```python
from build123d import *

# Parameters (mm, degrees)
BOSS_EXTRUDE6_DEPTH = 115
CUT_EXTRUDE5_START  = 2
SKETCH17_W          = 110
SKETCH17_H          = 71
CUT_EXTRUDE5_DEPTH  = 115
BOSS_EXTRUDE7_START = -12
BOSS_EXTRUDE7_DEPTH = 91
SKETCH22_R          = 3
SKETCH22_W          = 91
SKETCH22_H          = 3.970785373
CUT_EXTRUDE6_DEPTH  = 3.191306198
BOSS_EXTRUDE8_START = -12
SKETCH23_W          = 67.315835607
SKETCH23_H          = 18
BOSS_EXTRUDE8_DEPTH = 1
BOSS_EXTRUDE9_START = -12
SKETCH24_W          = 67.315835607
SKETCH24_H          = 18
BOSS_EXTRUDE9_DEPTH = 1
CUT_EXTRUDE7_DEPTH  = 1
CUT_EXTRUDE8_DEPTH  = 1


with BuildPart() as part:
    # Sketch16 → Boss-Extrude6 (new body)
    with BuildSketch(Plane(origin=(0, 0, 0), x_dir=(0, 0, -1), z_dir=(1, 0, 0))):
        Polygon((21.546513219, 40.639365956), (7.618622676, 40.639365956), (-0.073583226, 40.318426006), (-0.073583226, -0.191306198), (74.926416774, -0.191306198), (74.926416774, 34.808693802), (56.287613548, 38.312228243), (46.171210173, 39.731159859), (35.60256896, 40.205500696), (35.23833782, 40.205500696), align=None)
    extrude(amount=BOSS_EXTRUDE6_DEPTH)

    # Sketch17 → Cut-Extrude5 (cut)
    with BuildSketch(Plane(origin=(0, 0, 0), x_dir=(1, 0, 0), z_dir=(0, 1, 0)).offset(CUT_EXTRUDE5_START)):
        with Locations((57.5, 37.426416774)):
            Rectangle(SKETCH17_W, SKETCH17_H)
    extrude(amount=CUT_EXTRUDE5_DEPTH, mode=Mode.SUBTRACT)

    # Sketch21 → Boss-Extrude7 (add)
    with BuildSketch(Plane.ZY.offset(BOSS_EXTRUDE7_START)):
        with BuildLine():
            Line((-73.213037754, 2), (-73.213037754, 20))
            ThreePointArc((-73.213037754, 20), (-57.828004717, 3.773036878), (-40.805119951, 18.272518522))
            Line((-40.805119951, 18.272518522), (-38.305119951, 18.272518522))
            ThreePointArc((-38.305119951, 18.272518522), (-21.282235184, 3.773036878), (-5.897202147, 20))
            Line((-5.897202147, 20), (-5.897202147, 2))
            Line((-5.897202147, 2), (-73.213037754, 2))
        make_face()
    extrude(amount=-BOSS_EXTRUDE7_DEPTH)

    # Sketch22 → Cut-Extrude6 (cut, through all)
    with BuildSketch(Plane(origin=(0, 2, 0), x_dir=(1, 0, 0), z_dir=(0, 1, 0))):
        with Locations((7, 69.426416774)):
            Circle(SKETCH22_R)
        with Locations((108, 69.426416774)):
            Circle(SKETCH22_R)
        with Locations((108, 5.426416774)):
            Circle(SKETCH22_R)
        with Locations((7, 5.426416774)):
            Circle(SKETCH22_R)
        with Locations((57.5, 3.911809461)):
            Rectangle(SKETCH22_W, SKETCH22_H)
    extrude(amount=-CUT_EXTRUDE6_DEPTH, mode=Mode.SUBTRACT)

    # Sketch23 → Boss-Extrude8 (add)
    with BuildSketch(Plane.ZY.offset(BOSS_EXTRUDE8_START)):
        with Locations((-39.55511995, 11)):
            Rectangle(SKETCH23_W, SKETCH23_H)
    extrude(amount=BOSS_EXTRUDE8_DEPTH)

    # Sketch24 → Boss-Extrude9 (add)
    with BuildSketch(Plane(origin=(115, 0, 0), x_dir=(0, 0, -1), z_dir=(1, 0, 0)).offset(BOSS_EXTRUDE9_START)):
        with Locations((39.55511995, 11)):
            Rectangle(SKETCH24_W, SKETCH24_H)
    extrude(amount=BOSS_EXTRUDE9_DEPTH)

    # Sketch25 → Cut-Extrude7 (cut)
    with BuildSketch(Plane.ZY.offset(-11)):
        with BuildLine():
            Line((-68.205119951, 20), (-45.805119951, 20))
            ThreePointArc((-45.805119951, 20), (-57.005119951, 8.8), (-68.205119951, 20))
        make_face()
        with BuildLine():
            Line((-33.305119951, 20), (-10.905119951, 20))
            ThreePointArc((-10.905119951, 20), (-22.105119951, 8.8), (-33.305119951, 20))
        make_face()
    extrude(amount=-CUT_EXTRUDE7_DEPTH, mode=Mode.SUBTRACT)

    # Sketch26 → Cut-Extrude8 (cut)
    with BuildSketch(Plane(origin=(104, 0, 0), x_dir=(0, 0, -1), z_dir=(1, 0, 0))):
        with BuildLine():
            Line((10.905119951, 20), (33.305119951, 20))
            ThreePointArc((33.305119951, 20), (22.105119951, 8.8), (10.905119951, 20))
        make_face()
        with BuildLine():
            Line((45.805119951, 20), (68.205119951, 20))
            ThreePointArc((68.205119951, 20), (57.005119951, 8.8), (45.805119951, 20))
        make_face()
    extrude(amount=-CUT_EXTRUDE8_DEPTH, mode=Mode.SUBTRACT)


solid = part.part
```
Read the model definition and answer for the solid it produces. Units are mm, in the model's axes. A direction names the side the tool comes from. Coordinates: 2 decimals unless noted, no trailing zeros. Write each loop counter-clockwise with the first axis right and the second up, starting at its lowest first coordinate (ties: lowest second). Pieces come first, ordered by that corner, then holes. Notation, with made-up numbers: (9, 46) - (31, 46) arc R27 cw to (31, 68) - close; hole circle Ø1 at (39, 34). An arc over 180 degrees is marked (long way). Answer as a JSON object with one key per item and string values. Group by question number.
1. A cutting plane is placed at A-A (x = 7). Determine the outline of the cut face in (y, z).
2. A cutting plane is placed at B-B (y = 23.5). Determine the outline of the cut face in (x, z).
3. Each of these flat-tipped pins is pushed along its axis until it touches: P1, Ø8, axis at y = 26.5, z = -54.5, coming from the -X side; P2, Ø4, axis at x = 41.5, z = -38.5, coming from the +Y side; P3, Ø0.5, axis at x = 11.5, z = -8, coming from the +Y side; P4, Ø8, axis at x = 68.5, z = -52.5, coming from the +Y side. Where does it stop, or does it pass through?
4. The mould has two halves that part along Z. Classify faces 4 (the flat face through (113.73, 39.01, -51.3)), 5 (the flat face through (0, 21, -37)), 6 (the flat face through (109, 2, -38)): +Z half, -Z half, draft (parallel to the pull), parting line (faces both ways), or undercut.
5. Which of the six approach directions +Z, -Z, +X, -X, +Y, -Y give full straight-line access (tool end or side, diameter ignored) to faces 1 (the flat face through (12, 1, -4)), 2 (the cylindrical face through (103.507, 8.803, -22.351)), 3 (the flat face through (57, 17, -74.926))?
6. A cutting plane is placed at C-C (z = -31). Determine the outline of the cut face in (x, y).
7. Consider L1, parallel to X at y = 12.5, z = -32.5; L2, parallel to Z at x = 108, y = 1.2; L3, parallel to X at y = 4.5, z = -7. Determine where each line is inside the solid, lowest interval first. Write a range as [from, to].
8. A cutting plane is placed at D-D (y = 7.5). Determine the outline of the cut face in (x, z).
Worked out:
{
 "1": {"outline": "(-0.19, -74.93) - (34.81, -74.93) - (35.18, -72.93) - (2, -72.93) - (2, -72.43) - (-0.19, -72.43) - close; (-0.19, -66.43) - (2, -66.43) - (2, -8.43) - (-0.19, -8.43) - close; (-0.19, -2.43) - (2, -2.43) - (2, -1.93) - (40.4, -1.93) - (40.32, 0.07) - (-0.19, 0.07) - close"},
 "2": {"outline": "(0, -74.93) - (115, -74.93) - (115, 0.07) - (0, 0.07) - close; hole (2.5, -72.93) - (112.5, -72.93) - (112.5, -1.93) - (2.5, -1.93) - close"},
 "3": {"P1": "stops at x = 0", "P2": "stops at y = 18.27", "P3": "stops at y = 20", "P4": "stops at y = 6.13"},
 "4": {"face 4": "-Z half", "face 5": "draft", "face 6": "undercut"},
 "5": {"face 1": "+Y, -Y", "face 2": "+Y", "face 3": "-Z, +X, -X, +Y, -Y"},
 "6": {"outline": "(0, -0.19) - (115, -0.19) - (115, 40.34) - (112.5, 40.34) - (112.5, 2) - (104, 2) - (104, 13.19) - (103, 13.19) - (103, 6.37) - (12, 6.37) - (12, 13.19) - (11, 13.19) - (11, 2) - (2.5, 2) - (2.5, 40.34) - (0, 40.34) - close"},
 "7": {"L1": "x = [0, 2.5], [11, 12], [103, 104], [112.5, 115]", "L2": "z = [-74.93, -72.43], [-66.43, -8.43], [-2.43, 0.07]", "L3": "x = [0, 2.5], [11, 104], [112.5, 115]"},
 "8": {"outline": "(0, -74.93) - (115, -74.93) - (115, 0.07) - (0, 0.07) - close; hole (2.5, -72.93) - (11, -72.93) - (11, -5.9) - (104, -5.9) - (104, -72.93) - (112.5, -72.93) - (112.5, -1.93) - (2.5, -1.93) - close; hole (12, -67.35) - (103, -67.35) - (103, -46.58) - (12, -46.58) - close; hole (12, -32.53) - (103, -32.53) - (103, -11.76) - (12, -11.76) - close"}
}
